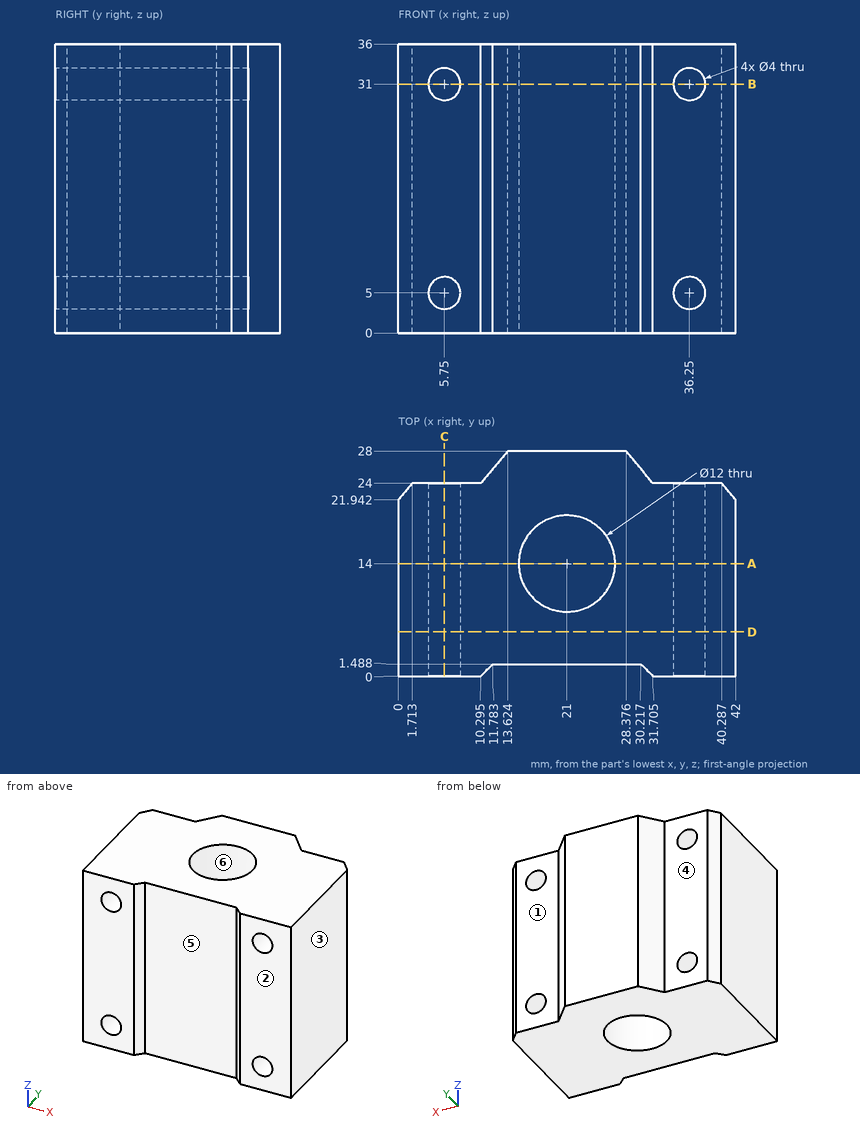
Verification items for this drawing (mm, ordinates from the low corner). A direction names the side the tool comes from. Give positions to 0.01 mm unless a question says otherwise; leave off trailing zeros. Loops run counter-clockwise (first coordinate to the right, second up) from the corner with the lowest first, then second, coordinate; pieces in that order, holes last. Notation, with made-up numbers: M -31.75,67 L -19.75,67 A33 cw -19.75,95 Z; hole C -36.75,-2 d8. An arc over 180 degrees is marked long. Write each question's results on one line, items separated by ' | '.
1) Thickness scan on line 1 (Z direction, x = 5.75, y = 6.5); line 2 (Z direction, x = 6.5, y = 14.5) (1 decimal); line 3 (Y direction, x = 21, z = 21). Record the ranges inside material, lowest first.
Answers follow:
line 1: 0 to 3, 7 to 29, 33 to 36 | line 2: 0 to 3.1, 6.9 to 29.1, 32.9 to 36 | line 3: 1.49 to 8, 20 to 28
2) Section check D-D, the plane y = 5.5. Record the boundary of the cut face in (x, z).
Answers follow:
outline: M 0,0 L 42,0 L 42,36 L 0,36 Z; hole C 5.75,5 d4; hole C 5.75,31 d4; hole C 36.25,5 d4; hole C 36.25,31 d4
3) Gauge pin test, flat ends, axial feed: pin 1 (5 mm diameter, centred on x = 27.5, z = 30, fed in from -Y); pin 2 (4.5 mm diameter, centred on x = 38, z = 24, fed in from +Y); pin 3 (10 mm diameter, centred on x = 35.5, z = 25, fed in from +Y). Record the tip position at first contact, or that the pin passes through.
Answers follow:
pin 1: y = 1.49 | pin 2: y = 24 | pin 3: y = 25.45
4) Section check A-A, the plane y = 14. Record the boundary of the cut face in (x, z), plus the area to 3 significant figures.
Answers follow:
outline: M 0,0 L 15,0 L 15,36 L 0,36 Z; M 27,0 L 42,0 L 42,36 L 27,36 Z; hole C 5.75,5 d4; hole C 5.75,31 d4; hole C 36.25,5 d4; hole C 36.25,31 d4 | area: 1,030 mm2
5) Release check for a two-part mould opening along Y. For the marked faces 3, 4, 5 and 6 record: +Y half, -Y half, draft (parallel to the pull), parting line (faces both ways), or undercut.
Answers follow:
face 3: draft | face 4: +Y half | face 5: -Y half | face 6: undercut
6) Tool access check on the marked faces 1 and 2. Record the directions out of +Z, -Z, +X, -X, +Y, -Y that give a thin tool (end or side, any length) a straight path to the whole face; none if there is none.
Answers follow:
face 1: +Z, -Z, +X, +Y | face 2: +Z, -Z, +X, -X, -Y
7) Section check B-B, the plane z = 31. Count the separate pieces of the cut face and the enclosed holes in it, plus the area to 3 significant figures.
Answers follow:
separate pieces: 3 | enclosed holes: 1 | area: 742 mm2
8) Section check C-C, the plane x = 5.75. Record the boundary of the cut face in (y, z).
Answers follow:
outline: M 0,0 L 24,0 L 24,3 L 0,3 Z; M 0,7 L 24,7 L 24,29 L 0,29 Z; M 0,33 L 24,33 L 24,36 L 0,36 Z
